from build123d import *

# Parameters (mm, degrees)
EXTRUDE_1_DEPTH = 4
FILLET_1_R      = 5
FILLET_2_R      = 10


with BuildPart() as part:
    # Эскиз1 → Бобышка-Вытянуть1 (new body)
    with BuildSketch(Plane.XY):
        Polygon((0, 0), (0, 125), (10, 125), (200, -140.041507642), align=None)
    extrude(amount=EXTRUDE_1_DEPTH)

    # Скругление1
    fillet_1_edges = [part.edges().sort_by_distance(p)[0] for p in [
        (200, -140.041507642, 2),
    ]]
    fillet(fillet_1_edges, radius=FILLET_1_R)

    # Скругление2
    fillet_2_edges = [part.edges().sort_by_distance(p)[0] for p in [
        (10, 125, 2),
    ]]
    fillet(fillet_2_edges, radius=FILLET_2_R)


solid = part.part
CAD build for the part. Positions are in the model's coordinates, mm. Give positions to 0.01 mm unless a question says otherwise; leave off trailing zeros. Loops run counter-clockwise (first coordinate to the right, second up) from the corner with the lowest first, then second, coordinate; pieces in that order, holes last. Notation, with made-up numbers: M -11.5,-19.75 L 25.5,-19.75 A12 cw 25.5,1.25 Z; hole C 57,-10 d10. An arc over 180 degrees is marked long. Answer in a Markdown table with one row per item. Add a question column.
Item 1: Band-saw the part on A-A on z = 2.65. Give the cut face in (x, y).
Item 2: Probe probe 1 along X at (y, z) = (45, 3.2); probe 2 along Y at (x, z) = (68.5, 1); probe 3 along X at (y, z) = (-113, 3.5). List the from-to ranges inside material, lowest first.
Item 3: Band-saw the part on C-C on x = 57.5. Give the cut face in (y, z).
Item 4: Band-saw the part on B-B on y = -84. Give the cut face in (x, z).
Item 5: Drop flat-ended pins along their axis: P1, Ø1, axis at y = -12.5, z = 1.5, coming from the +X side; P2, Ø2, axis at x = 123, z = 2, coming from the -Y side. Give the stop position or say it passes through.
Reply:
| question | item | result |
|---|---|---|
| 1 | outline | M 0,0 L 175.99,-123.23 A5 ccw 182.93,-116.22 L 12.99,120.83 A10 ccw 4.86,125 L 0,125 Z |
| 2 | probe 1 | x = 0 to 67.35 |
| 2 | probe 2 | y = -47.96 to 43.4 |
| 2 | probe 3 | x = 161.38 to 180.61 |
| 3 | outline | M -40.26,0 L 58.74,0 L 58.74,4 L -40.26,4 Z |
| 4 | outline | M 119.96,0 L 159.83,0 L 159.83,4 L 119.96,4 Z |
| 5 | P1 | stops at x = 108.93 |
| 5 | P2 | stops at y = -86.83 |
